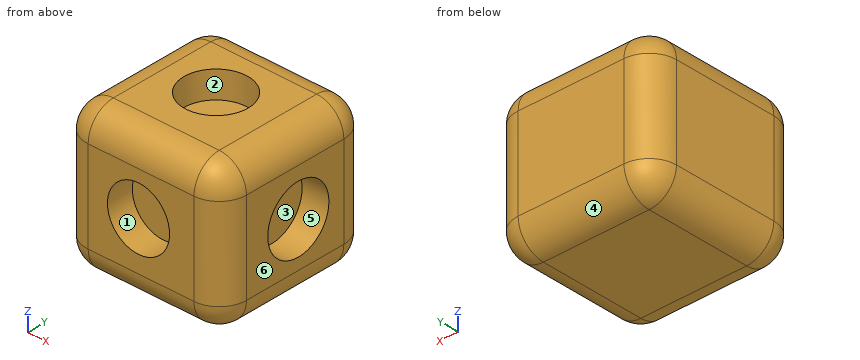
from build123d import *

# Parameters (mm, degrees)
F0_W     = 151.631288
F0_H     = 150.920756
F1_DEPTH = 137.922
F2_R     = 25.75483
F3_R     = 30.269305
F4_DEPTH = 25.4
F5_R     = 29.389096
F6_DEPTH = 25.4
F7_R     = 31.234323
F8_DEPTH = 25.4


with BuildPart() as f1:
    # F0 (on Top) → F1 (new body)
    with BuildSketch(Plane.XY):
        with Locations((0.510808, -0.572886)):
            Rectangle(F0_W, F0_H)
    extrude(amount=F1_DEPTH)

    # F2
    f2_edges = [f1.edges().sort_by_distance(p)[0] for p in [
        (0.510808, 74.887492, 137.922),
        (-75.304836, -0.572886, 137.922),
        (0.510808, -76.033264, 137.922),
        (76.326452, -0.572886, 137.922),
        (76.326452, -76.033264, 68.961),
        (76.326452, 74.887492, 68.961),
        (76.326452, -0.572886, 0),
        (-75.304836, -76.033264, 68.961),
        (0.510808, -76.033264, 0),
        (-75.304836, 74.887492, 68.961),
        (-75.304836, -0.572886, 0),
        (0.510808, 74.887492, 0),
    ]]
    fillet(f2_edges, radius=F2_R)

    # F3 (on face) → F4 (cut)
    with BuildSketch(Plane.XY.offset(137.922)):
        with Locations((-2.210455, 3.441766)):
            Circle(F3_R)
    extrude(amount=-F4_DEPTH, mode=Mode.SUBTRACT)

    # F5 (on face) → F6 (cut)
    with BuildSketch(Plane.XZ.offset(76.033264)):
        with Locations((-1.93036, 71.224585)):
            Circle(F5_R)
    extrude(amount=-F6_DEPTH, mode=Mode.SUBTRACT)

    # F7 (on face) → F8 (cut)
    with BuildSketch(Plane.YZ.offset(76.326452)):
        with Locations((2.6777, 67.931794)):
            Circle(F7_R)
    extrude(amount=-F8_DEPTH, mode=Mode.SUBTRACT)


solid = f1.part
Work out the finished part from the listing and answer in its coordinate system (mm). Face numbers are marked on the shaded views. A direction names the side the tool comes from. Round coordinates to 2 decimals unless told otherwise and drop trailing zeros. Order: outer loops, then holes, each group sorted by start corner. A loop starts at its lowest first (then second) coordinate and runs counter-clockwise, first axis right, second up. Notation, with made-up numbers: M 67.5,87.25 L 110.5,87.25 A31 ccw 110.5,121.25 Z; hole C 36,-4.75 d8. An arc over 180 degrees is marked long. One line per item, written item: value.
Q1. Straight lines are drawn through the part: line 1 (Y direction, x = -14.5, z = 74.5); line 2 (X direction, y = 21, z = 117); line 3 (X direction, y = -9.5, z = 94). For each, find the intervals that lie inside material, in ascending order.
Derived:
line 1: -50.63 to 74.89
line 2: -74.85 to -26.87, 22.45 to 75.87
line 3: -75.3 to 50.93
Q2. Find section D-D on z = 31. Write down the section's boundary in (x, y).
Derived:
outline: M -75.3,-50.28 A25.75 ccw -49.55,-76.03 L 50.57,-76.03 A25.75 ccw 76.33,-50.28 L 76.33,49.13 A25.75 ccw 50.57,74.89 L -49.55,74.89 A25.75 ccw -75.3,49.13 Z
Q3. Find section C-C on z = 124. Write down the section's boundary in (x, y).
Derived:
outline: M -72.43,-50.28 A22.88 ccw -49.55,-73.15 L 50.57,-73.15 A22.88 ccw 73.45,-50.28 L 73.45,49.13 A22.88 ccw 50.57,72.01 L -49.55,72.01 A22.88 ccw -72.43,49.13 Z; hole C -2.21,3.44 d60.54
Q4. Determine the mould class of the marked faces 4, 5 and 6 for opening direction Z: released by +Z, released by -Z, zero draft, split by the parting line, or undercut.
Derived:
face 4: released by -Z
face 5: undercut
face 6: zero draft
Q5. Find section A-A on x = 31. Write down the section's boundary in (y, z).
Derived:
outline: M -76.03,25.75 A25.75 ccw -50.28,0 L 49.13,0 A25.75 ccw 74.89,25.75 L 74.89,112.17 A25.75 ccw 49.13,137.92 L -50.28,137.92 A25.75 ccw -76.03,112.17 Z
Q6. Find section B-B on y = -55. Write down the section's boundary in (x, z), then the cut area to 3 significant figures.
Derived:
outline: M -74.87,25.75 A25.32 ccw -49.55,0.44 L 50.57,0.44 A25.32 ccw 75.89,25.75 L 75.89,112.17 A25.32 ccw 50.57,137.49 L -49.55,137.49 A25.32 ccw -74.87,112.17 Z; hole C -1.93,71.22 d58.78
area: 17,400 mm²
Q7. For the marked faces 1, 2 and 3, determine the directions among +Z, -Z, +X, -X, +Y, -Y from which every point of the face is accessible in a straight line to the end or side of a thin tool.
Derived:
face 1: -Y
face 2: +Z
face 3: +X
Q8. Flat-ended cylindrical pins translate along their axes: pin 1 (1 mm diameter, centred on y = 9, z = 62, fed in from +X); pin 2 (5 mm diameter, centred on x = 22, z = 15, fed in from +Y); pin 3 (1 mm diameter, centred on y = -18.5, z = 23.5, fed in from +X). Find the tip coordinate at first contact, or state that the pin passes through.
Derived:
pin 1: x = 50.93
pin 2: y = 73.53
pin 3: x = 76.27
